Could you check a few things on this model? Use its own coordinates, in mm. Face numbers are marked on the shaded views. A direction names the side the tool comes from. Round coordinates to 2 decimals unless told otherwise and drop trailing zeros. Order: outer loops, then holes, each group sorted by start corner. A loop starts at its lowest first (then second) coordinate and runs counter-clockwise, first axis right, second up. Notation, with made-up numbers: (20, 72) - (49, 72) arc R15 cw to (49, 93) - close; hole circle Ø5 at (-31, 64.25). An arc over 180 degrees is marked (long way). Use one line per item in the form item = value.
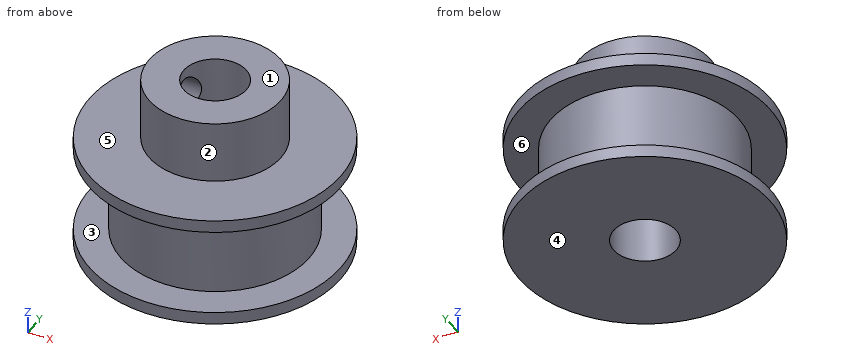
from build123d import *

# Parameters (mm, degrees)
ESQUISSE1_R             = 10
BOSS_EXTRU_1_DEPTH      = 9
ESQUISSE2_R             = 5.25
BOSS_EXTRU_2_DEPTH      = 5
ESQUISSE3_R             = 2.5
ENL_V_MAT_EXTRU_1_DEPTH = 20.899748742
ESQUISSE4_W             = 7
ESQUISSE4_H             = 2.5


# Read off the part's stored shape, not the designer's step: Dégagement M31
with BuildPart() as part:
    # Esquisse1 → Boss.-Extru.1 (new body)
    with BuildSketch(Plane.XY):
        Circle(ESQUISSE1_R)
    extrude(amount=BOSS_EXTRU_1_DEPTH)

    # Esquisse2 → Boss.-Extru.2 (add)
    with BuildSketch(Plane.XY.offset(9)):
        Circle(ESQUISSE2_R)
    extrude(amount=BOSS_EXTRU_2_DEPTH)

    # Esquisse3 → Enlèv. mat.-Extru.1 (cut, through all)
    with BuildSketch(Plane.XY.offset(14)):
        Circle(ESQUISSE3_R)
    extrude(amount=-ENL_V_MAT_EXTRU_1_DEPTH, mode=Mode.SUBTRACT)

    # Esquisse4 → Enlèvement de matière-Révolution1 (revolve, cut)
    with BuildSketch(Plane(origin=(0, 0, 0), x_dir=(0, 0, -1), z_dir=(1, 0, 0)), mode=Mode.PRIVATE) as enl_vement_de_mati_re_r_volution1_sk:
        with Locations((-4.5, 8.75)):
            Rectangle(ESQUISSE4_W, ESQUISSE4_H)
    revolve(enl_vement_de_mati_re_r_volution1_sk.sketch.rotate(Axis((0, 0, 0), (0, 0, 1)), 90), axis=Axis((0, 0, 0), (0, 0, 1)), mode=Mode.SUBTRACT)

    # Dégagement M31 outline → Dégagement M31 (revolve, cut)
    with BuildSketch(Plane.YX.offset(-11.551623765)):
        Polygon((1.6, -5.250016412), (1.6, -5.225), (1.6, -1.920645137), (0, -1.920645137), (0, -5.250016412), align=None)
        Polygon((1.625016412, -5.250016412), (1.599998144, -5.224998144), (1.6, -5.250016412), align=None)
    revolve(axis=Axis((0, 0, 11.551623765), (1, 0, 0)), mode=Mode.SUBTRACT)


solid = part.part
Item 1: Imagine slicing it at A-A on x = 0. Please give me the cut outline in (y, z).
Found:
outline = (-10, 0) - (-2.5, 0) - (-2.5, 14) - (-5.25, 14) - (-5.25, 9) - (-10, 9) - (-10, 8) - (-7.5, 8) - (-7.5, 1) - (-10, 1) - close; (2.5, 0) - (10, 0) - (10, 1) - (7.5, 1) - (7.5, 8) - (10, 8) - (10, 9) - (5.25, 9) - (5.25, 14) - (2.5, 14) - close
Item 2: I need wall thicknesses on L1, parallel to X at y = 0, z = 9.5; L2, parallel to Z at x = 0.75, y = -8; L3, parallel to Y at x = 0, z = 6.25. Which ranges of each line are inside material? Lowest first, please.
Found:
L1 = -5.25 to -2.5, 2.5 to 5.25
L2 = 0 to 1, 8 to 9
L3 = -7.5 to -2.5, 2.5 to 7.5
Item 3: For the marked faces 1, 2 and 3, which set-ups out of +Z, -Z, +X, -X, +Y, -Y let a thin tool reach every point of the face, with its end or its side?
Found:
face_1 = +Z, +X, -X, +Y, -Y
face_2 = +Z
face_3 = none
Item 4: If we mould it in two halves opening along Z, with no side actions, what happens to the marked faces 4, 5 and 6? For each: released by +Z, released by -Z, zero draft, split by the parting line, or undercut.
Found:
face_4 = released by -Z
face_5 = released by +Z
face_6 = undercut
Item 5: Imagine slicing it at D-D on x = -3.5. Please give me the cut outline in (y, z), plus the area to 3 significant figures.
Found:
outline = (-9.37, 0) - (9.37, 0) - (9.37, 1) - (6.63, 1) - (6.63, 8) - (9.37, 8) - (9.37, 9) - (3.91, 9) - (3.91, 14) - (-3.91, 14) - (-3.91, 9) - (-9.37, 9) - (-9.37, 8) - (-6.63, 8) - (-6.63, 1) - (-9.37, 1) - close; hole circle Ø3.2 at (0, 11.55)
area = 161 mm2
Item 6: Imagine slicing it at C-C on z = 2.75. Please give me the cut outline in (x, y), plus the area to 3 significant figures.
Found:
outline = circle Ø15 at (0, 0); hole circle Ø5 at (0, 0)
area = 157 mm2
Item 7: Imagine slicing it at B-B on y = 0. Please give me the cut outline in (x, z) (3 decimals), plus the area to 3 significant figures.
Found:
outline = (-10, 0) - (-2.5, 0) - (-2.5, 9.952) - (-5.225, 9.952) - (-5.25, 9.927) - (-5.25, 9) - (-10, 9) - (-10, 8) - (-7.5, 8) - (-7.5, 1) - (-10, 1) - close; (-5.25, 13.177) - (-5.225, 13.152) - (-2.5, 13.152) - (-2.5, 14) - (-5.25, 14) - close; (2.5, 0) - (10, 0) - (10, 1) - (7.5, 1) - (7.5, 8) - (10, 8) - (10, 9) - (5.25, 9) - (5.25, 14) - (2.5, 14) - close
area = 119 mm2
Item 8: Will these pins go through, and if not, where does the flat tip stop? P1, Ø5, axis at y = 6, z = 10, coming from the +X side; P2, Ø3, axis at y = 0, z = 11.55, coming from the +X side; P3, Ø6, axis at x = 6.5, z = 11.5, coming from the -Y side.
Found:
P1 = 9.29
P2 = 5.25
P3 = -8.75
